Design review of the part built by this model. Coordinates are the model's own, in mm. Coordinates: 2 decimals unless noted, no trailing zeros. Loops run counter-clockwise (first coordinate to the right, second up) from the corner with the lowest first, then second, coordinate; pieces in that order, holes last.
Q1. Add section B-B on z = -29. Give the boundary of the cut face in (x, y), and give its area (3 significant figures).
Q2. Wall thickness on probe 1 along X at (y, z) = (1.5, -40.5); probe 2 along Z at (x, y) = (63, 2); probe 3 along Z at (x, y) = (211.5, 1.25): over which ranges is each line inside the solid? List them lowest first.
Q3. Add section A-A on x = 247. Give the boundary of the cut face in (y, z), and give its area (3 significant figures).
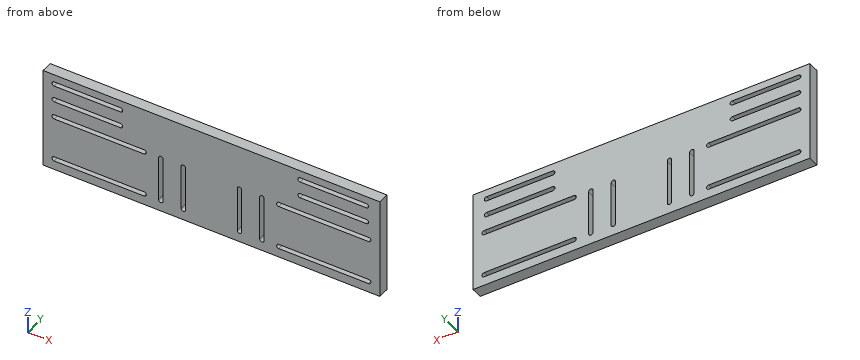
```python
from build123d import *

# Parameters (mm, degrees)
SKETCH1_W           = 300
SKETCH1_H           = 30
BOSS_EXTRUDE1_DEPTH = 10
SKETCH2_W           = 300
SKETCH2_H           = 10
BOSS_EXTRUDE2_DEPTH = 60
CUT_EXTRUDE1_DEPTH  = 307.1045573


with BuildPart() as part:
    # Sketch1 → Boss-Extrude1 (new body)
    with BuildSketch(Plane(origin=(0, 0, 0), x_dir=(1, 0, 0), z_dir=(0, 1, 0))):
        with Locations((150, -15)):
            Rectangle(SKETCH1_W, SKETCH1_H)
        with BuildLine():
            Line((68.977444605, -8.309450677), (10, -8.309450677))
            ThreePointArc((10, -8.309450677), (8, -6.309450677), (10, -4.309450677))
            Line((10, -4.309450677), (68.977444605, -4.309450677))
            ThreePointArc((68.977444605, -4.309450677), (70.977444605, -6.309450677), (68.977444605, -8.309450677))
        make_face(mode=Mode.SUBTRACT)
        with BuildLine():
            Line((68.977444605, -23.309450677), (10, -23.309450677))
            ThreePointArc((10, -23.309450677), (8, -21.309450677), (10, -19.309450677))
            Line((10, -19.309450677), (68.977444605, -19.309450677))
            ThreePointArc((68.977444605, -19.309450677), (70.977444605, -21.309450677), (68.977444605, -23.309450677))
        make_face(mode=Mode.SUBTRACT)
        with BuildLine():
            Line((228.977444605, -23.309450677), (287.95488921, -23.309450677))
            ThreePointArc((287.95488921, -23.309450677), (289.95488921, -21.309450677), (287.95488921, -19.309450677))
            Line((287.95488921, -19.309450677), (228.977444605, -19.309450677))
            ThreePointArc((228.977444605, -19.309450677), (226.977444605, -21.309450677), (228.977444605, -23.309450677))
        make_face(mode=Mode.SUBTRACT)
        with BuildLine():
            Line((228.977444605, -8.309450677), (287.95488921, -8.309450677))
            ThreePointArc((287.95488921, -8.309450677), (289.95488921, -6.309450677), (287.95488921, -4.309450677))
            Line((287.95488921, -4.309450677), (228.977444605, -4.309450677))
            ThreePointArc((228.977444605, -4.309450677), (226.977444605, -6.309450677), (228.977444605, -8.309450677))
        make_face(mode=Mode.SUBTRACT)
    extrude(amount=BOSS_EXTRUDE1_DEPTH)

    # Sketch2 → Boss-Extrude2 (add)
    with BuildSketch(Plane(origin=(0, 0, 0), x_dir=(-1, 0, 0), z_dir=(0, 0, -1))):
        with Locations((-150, 5)):
            Rectangle(SKETCH2_W, SKETCH2_H)
    extrude(amount=BOSS_EXTRUDE2_DEPTH)

    # Sketch3 → Cut-Extrude1 (cut, through all)
    with BuildSketch(Plane(origin=(0, 10, 0), x_dir=(1, 0, 0), z_dir=(0, 1, 0))):
        with BuildLine():
            Line((10, 52), (90, 52))
            ThreePointArc((90, 52), (92, 50), (90, 48))
            Line((90, 48), (10, 48))
            ThreePointArc((10, 48), (8, 50), (10, 52))
        make_face()
        with BuildLine():
            Line((10, 12), (90, 12))
            ThreePointArc((90, 12), (92, 10), (90, 8))
            Line((90, 8), (10, 8))
            ThreePointArc((10, 8), (8, 10), (10, 12))
        make_face()
        with BuildLine():
            Line((127, 50), (127, 10))
            ThreePointArc((127, 10), (125, 8), (123, 10))
            Line((123, 10), (123, 50))
            ThreePointArc((123, 50), (125, 52), (127, 50))
        make_face()
        with BuildLine():
            Line((107, 50), (107, 10))
            ThreePointArc((107, 10), (105, 8), (103, 10))
            Line((103, 10), (103, 50))
            ThreePointArc((103, 50), (105, 52), (107, 50))
        make_face()
        with BuildLine():
            Line((290, 52), (210, 52))
            ThreePointArc((210, 52), (208, 50), (210, 48))
            Line((210, 48), (290, 48))
            ThreePointArc((290, 48), (292, 50), (290, 52))
        make_face()
        with BuildLine():
            Line((290, 12), (210, 12))
            ThreePointArc((210, 12), (208, 10), (210, 8))
            Line((210, 8), (290, 8))
            ThreePointArc((290, 8), (292, 10), (290, 12))
        make_face()
        with BuildLine():
            Line((173, 50), (173, 10))
            ThreePointArc((173, 10), (175, 8), (177, 10))
            Line((177, 10), (177, 50))
            ThreePointArc((177, 50), (175, 52), (173, 50))
        make_face()
        with BuildLine():
            Line((193, 50), (193, 10))
            ThreePointArc((193, 10), (195, 8), (197, 10))
            Line((197, 10), (197, 50))
            ThreePointArc((197, 50), (195, 52), (193, 50))
        make_face()
    extrude(amount=-CUT_EXTRUDE1_DEPTH, mode=Mode.SUBTRACT)


solid = part.part
```
Entries:
1. outline: (0, 0) - (103, 0) - (103, 10) - (0, 10) - close; (107, 0) - (123, 0) - (123, 10) - (107, 10) - close; (127, 0) - (173, 0) - (173, 10) - (127, 10) - close; (177, 0) - (193, 0) - (193, 10) - (177, 10) - close; (197, 0) - (300, 0) - (300, 10) - (197, 10) - close
1. area: 2,840 mm2
2. probe 1: x = 0 to 103, 107 to 123, 127 to 173, 177 to 193, 197 to 300
2. probe 2: z = -60 to -52, -48 to -12, -8 to 4.31, 8.31 to 19.31, 23.31 to 30
2. probe 3: z = -60 to -52, -48 to -12, -8 to 30
3. outline: (0, -60) - (10, -60) - (10, -52) - (0, -52) - close; (0, -48) - (10, -48) - (10, -12) - (0, -12) - close; (0, -8) - (10, -8) - (10, 4.31) - (0, 4.31) - close; (0, 8.31) - (10, 8.31) - (10, 19.31) - (0, 19.31) - close; (0, 23.31) - (10, 23.31) - (10, 30) - (0, 30) - close
3. area: 740 mm2
